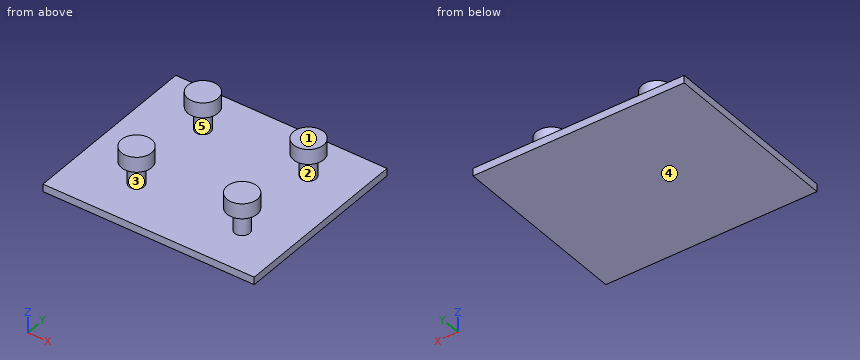
```python
from build123d import *

# Parameters (mm, degrees)
F1_START = 25.4
F0_R     = 12.7
F0_R_2   = 6.35
F1_DEPTH = 12.7
F2_DEPTH = 25.4
F0_W     = 177.8
F0_H     = 152.4
F3_DEPTH = 6.35


with BuildPart() as f1:
    # F0 (on Top) → F1 (new body)
    with BuildSketch(Plane.XY.offset(F1_START)):
        with Locations((-25.4, 38.1)):
            Circle(F0_R)
        with Locations((-25.4, 38.1)):
            Circle(F0_R_2, mode=Mode.SUBTRACT)
        with Locations((-25.4, 38.1)):
            Circle(F0_R_2)
    extrude(amount=F1_DEPTH)

    # F0 (on Top) → F2, piece 2 (join)
    with BuildSketch(Plane.XY):
        with Locations((-25.4, 38.1)):
            Circle(F0_R_2)
    extrude(amount=F2_DEPTH)



with BuildPart() as f1b:
    # F0 (on Top) → F1, piece 2 (new body)
    with BuildSketch(Plane.XY.offset(F1_START)):
        with Locations((63.5, 38.1)):
            Circle(F0_R)
        with Locations((63.5, 38.1)):
            Circle(F0_R_2, mode=Mode.SUBTRACT)
        with Locations((63.5, 38.1)):
            Circle(F0_R_2)
    extrude(amount=F1_DEPTH)

    # F0 (on Top) → F2 (join)
    with BuildSketch(Plane.XY):
        with Locations((63.5, 38.1)):
            Circle(F0_R_2)
    extrude(amount=F2_DEPTH)


with BuildPart() as f1c:
    # F0 (on Top) → F1, piece 3 (new body)
    with BuildSketch(Plane.XY.offset(F1_START)):
        with Locations((-25.4, -38.1)):
            Circle(F0_R)
        with Locations((-25.4, -38.1)):
            Circle(F0_R_2, mode=Mode.SUBTRACT)
        with Locations((-25.4, -38.1)):
            Circle(F0_R_2)
    extrude(amount=F1_DEPTH)

    # F0 (on Top) → F2, piece 3 (join)
    with BuildSketch(Plane.XY):
        with Locations((-25.4, -38.1)):
            Circle(F0_R_2)
    extrude(amount=F2_DEPTH)


with BuildPart() as f1d:
    # F0 (on Top) → F1, piece 4 (new body)
    with BuildSketch(Plane.XY.offset(F1_START)):
        with Locations((63.5, -38.1)):
            Circle(F0_R)
        with Locations((63.5, -38.1)):
            Circle(F0_R_2, mode=Mode.SUBTRACT)
        with Locations((63.5, -38.1)):
            Circle(F0_R_2)
    extrude(amount=F1_DEPTH)

    # F0 (on Top) → F2, piece 4 (join)
    with BuildSketch(Plane.XY):
        with Locations((63.5, -38.1)):
            Circle(F0_R_2)
    extrude(amount=F2_DEPTH)


with BuildPart() as f1_1:
    add(f1.part)

    add(f1b.part)  # F3 merges F1b

    add(f1c.part)  # F3 merges F1c

    add(f1d.part)  # F3 merges F1d
    # F0 (on Top) → F3 (join)
    with BuildSketch(Plane.XY):
        with Locations((12.7, 0)):
            Rectangle(F0_W, F0_H)
        with Locations((-25.4, -38.1)):
            Circle(F0_R, mode=Mode.SUBTRACT)
        with Locations((63.5, -38.1)):
            Circle(F0_R, mode=Mode.SUBTRACT)
        with Locations((-25.4, 38.1)):
            Circle(F0_R, mode=Mode.SUBTRACT)
        with Locations((63.5, 38.1)):
            Circle(F0_R, mode=Mode.SUBTRACT)
        with Locations((63.5, 38.1)):
            Circle(F0_R)
        with Locations((63.5, 38.1)):
            Circle(F0_R_2, mode=Mode.SUBTRACT)
        with Locations((-25.4, 38.1)):
            Circle(F0_R)
        with Locations((-25.4, 38.1)):
            Circle(F0_R_2, mode=Mode.SUBTRACT)
        with Locations((-25.4, -38.1)):
            Circle(F0_R)
        with Locations((-25.4, -38.1)):
            Circle(F0_R_2, mode=Mode.SUBTRACT)
        with Locations((63.5, -38.1)):
            Circle(F0_R)
        with Locations((63.5, -38.1)):
            Circle(F0_R_2, mode=Mode.SUBTRACT)
    extrude(amount=F3_DEPTH)


solid = f1_1.part
```
Could you check a few things on this model? Use its own coordinates, in mm. Face numbers are marked on the shaded views. A direction names the side the tool comes from. Give positions to 0.01 mm unless a question says otherwise; leave off trailing zeros. Loops run counter-clockwise (first coordinate to the right, second up) from the corner with the lowest first, then second, coordinate; pieces in that order, holes last. Notation, with made-up numbers: (80, 66) - (94, 66) arc R26 ccw to (94, 93) - close; hole circle Ø5 at (19, 65). An arc over 180 degrees is marked (long way). Use one line per item in the form item = value.
1. I want a section at A-A (z = 34). Please give me the cut outline in (x, y).
Response values:
outline = circle Ø25.4 at (-25.4, -38.1); circle Ø25.4 at (-25.4, 38.1); circle Ø25.4 at (63.5, -38.1); circle Ø25.4 at (63.5, 38.1)
2. I need wall thicknesses on probe 1 along Z at (x, y) = (43.5, -46); probe 2 along X at (y, z) = (48, 34); probe 3 along Y at (x, z) = (-36.5, 30.5). Which ranges of each line are inside material? Lowest first, please.
Response values:
probe_1 = 0 to 6.35
probe_2 = -33.35 to -17.45, 55.55 to 71.45
probe_3 = -44.27 to -31.93, 31.93 to 44.27
3. On a 3-axis mill with a long thin cutter (end or side, diameter ignored), from which of +Z, -Z, +X, -X, +Y, -Y can I reach the whole of each face in a straight line? I mean the marked faces 1 and 2. Say none if no direction works.
Response values:
face_1 = +Z, +X, -X, +Y, -Y
face_2 = none
4. I'm going to push flat-ended pins straight in: pin 1 Ø12 at (y, z) = (-23.5, 34) entering from +X; pin 2 Ø2 at (y, z) = (30, 27.5) entering from +X; pin 3 Ø12 at (x, z) = (63, 28) entering from -Y. Where does each tip first touch, or does it pass through?
Response values:
pin_1 = 72.85
pin_2 = 74.03
pin_3 = -50.8
5. I want a section at B-B (y = 38.1). Please give me the cut outline in (x, z).
Response values:
outline = (-76.2, 0) - (101.6, 0) - (101.6, 6.35) - (69.85, 6.35) - (69.85, 25.4) - (76.2, 25.4) - (76.2, 38.1) - (50.8, 38.1) - (50.8, 25.4) - (57.15, 25.4) - (57.15, 6.35) - (-19.05, 6.35) - (-19.05, 25.4) - (-12.7, 25.4) - (-12.7, 38.1) - (-38.1, 38.1) - (-38.1, 25.4) - (-31.75, 25.4) - (-31.75, 6.35) - (-76.2, 6.35) - close
6. Thinking about a two-plate mould opening in Y: for the marked faces 3, 4 and 5, which applies, released by +Y, released by -Y, zero draft, split by the parting line, or undercut?
Response values:
face_3 = undercut
face_4 = zero draft
face_5 = undercut
7. I want a section at D-D (z = 15). Please give me the cut outline in (x, y), and give its area (3 significant figures).
Response values:
outline = circle Ø12.7 at (-25.4, -38.1); circle Ø12.7 at (-25.4, 38.1); circle Ø12.7 at (63.5, -38.1); circle Ø12.7 at (63.5, 38.1)
area = 507 mm²
8. I want a section at C-C (x = -25.4). Please give me the cut outline in (y, z), and give its area (3 significant figures).
Response values:
outline = (-76.2, 0) - (76.2, 0) - (76.2, 6.35) - (44.45, 6.35) - (44.45, 25.4) - (50.8, 25.4) - (50.8, 38.1) - (25.4, 38.1) - (25.4, 25.4) - (31.75, 25.4) - (31.75, 6.35) - (-31.75, 6.35) - (-31.75, 25.4) - (-25.4, 25.4) - (-25.4, 38.1) - (-50.8, 38.1) - (-50.8, 25.4) - (-44.45, 25.4) - (-44.45, 6.35) - (-76.2, 6.35) - close
area = 2,100 mm²
